Part print with two shaded views. Sizes in mm from the minimum x, y, z corner. A direction names the side the tool comes from. Round coordinates to 2 decimals unless told otherwise and drop trailing zeros. Order: outer loops, then holes, each group sorted by start corner. A loop starts at its lowest first (then second) coordinate and runs counter-clockwise, first axis right, second up. Notation, with made-up numbers: (70.25, -28) -> (99.25, -28) arc R17 cw to (99.25, 2) -> close; hole circle Ø6 at (-6, 6.5). An arc over 180 degrees is marked (long way). Put each result on its own line as item: value. Start each with the question number.
Q1. Probe L1, parallel to Z at x = 44, y = 23 (1 decimal); L2, parallel to X at y = 11, z = 23.5 (1 decimal); L3, parallel to X at y = 17, z = 90. List the from-to ranges inside material, lowest first.
Q2. Cut at C-C, the plane x = 67.5. List the corners of the cut face in (y, z).
Q3. Pull direction Z, two halves, no side cores. Call the marked faces 1, 2 and 3: released by +Z, released by -Z, zero draft, split by the parting line, or undercut.
Q4. Cut at B-B, the plane z = 66. List the corners of the cut face in (x, y), and give its area (3 significant figures).
Q5. Cut at A-A, the plane y = 2.25. List the corners of the cut face in (x, z) (1 decimal), and give its area (3 significant figures).
Q6. Flat gauge pins, fed straight in: P1, Ø2, axis at x = 30.5, y = 12, coming from the +Z side; P2, Ø8, axis at y = 11.5, z = 25.5, coming from the +X side; P3, Ø5.5, axis at x = 64, y = 11, coming from the -Z side. Where does each tip first touch, or does it go through?
Q7. 3-axis set-ups, long thin cutter, end or side, ignore diameter. For the marked faces 4, 5 and 6: which of +Z, -Z, +X, -X, +Y, -Y reach the whole face in a straight line?
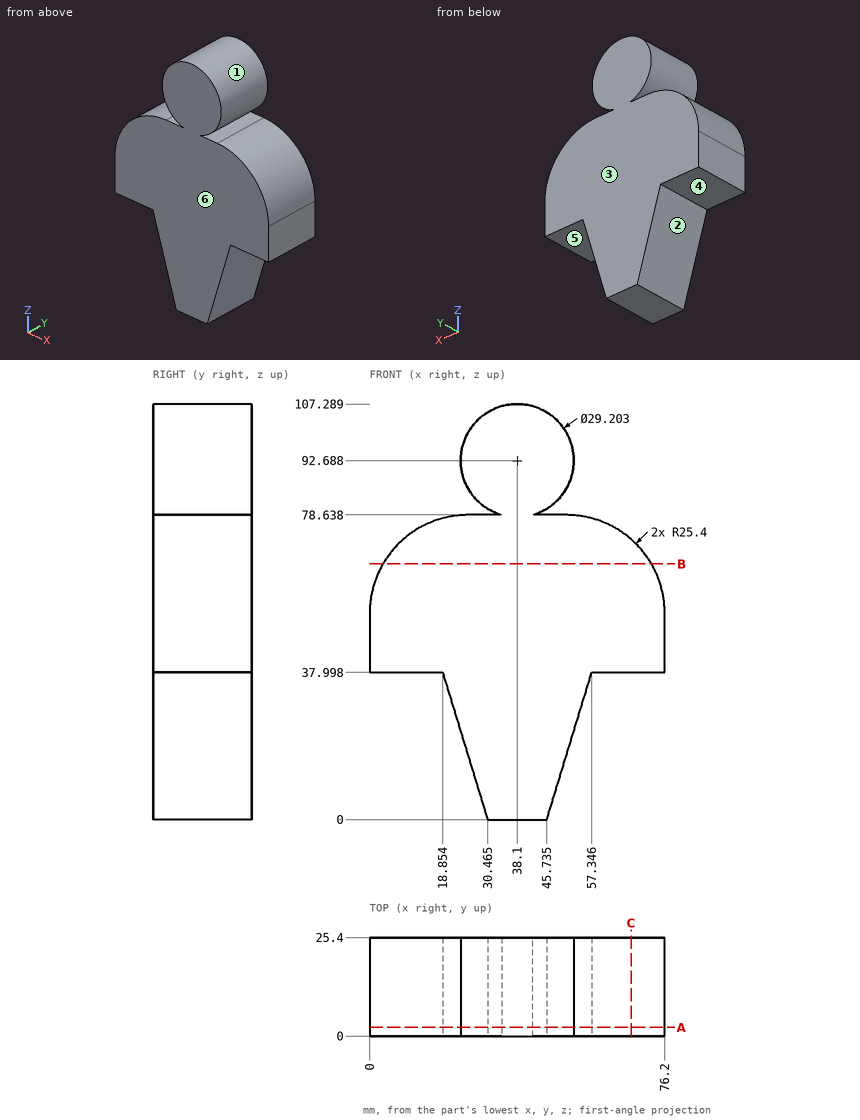
Ans:
1. L1: z = 0 to 78.6, 79.3 to 106
1. L2: x = 23.3 to 52.9
1. L3: x = 23.75 to 52.45
2. outline: (0, 38) -> (25.4, 38) -> (25.4, 72.38) -> (0, 72.38) -> close
3. face 1: undercut
3. face 2: released by -Z
3. face 3: zero draft
4. outline: (3.44, 0) -> (72.76, 0) -> (72.76, 25.4) -> (3.44, 25.4) -> close
4. area: 1,760 mm^2
5. outline: (0, 38) -> (18.9, 38) -> (30.5, 0) -> (45.7, 0) -> (57.3, 38) -> (76.2, 38) -> (76.2, 53.2) arc R25.4 ccw to (50.8, 78.6) -> (42.1, 78.6) arc R14.6 ccw (long way) to (34.1, 78.6) -> (25.4, 78.6) arc R25.4 ccw to (0, 53.2) -> close
5. area: 4,510 mm^2
6. P1: stops at z = 105.71
6. P2: stops at x = 54.75
6. P3: stops at z = 38
7. face 4: -Z, -X, +Y, -Y
7. face 5: -Z, +X, +Y, -Y
7. face 6: +Z, -Z, +X, -X, -Y
